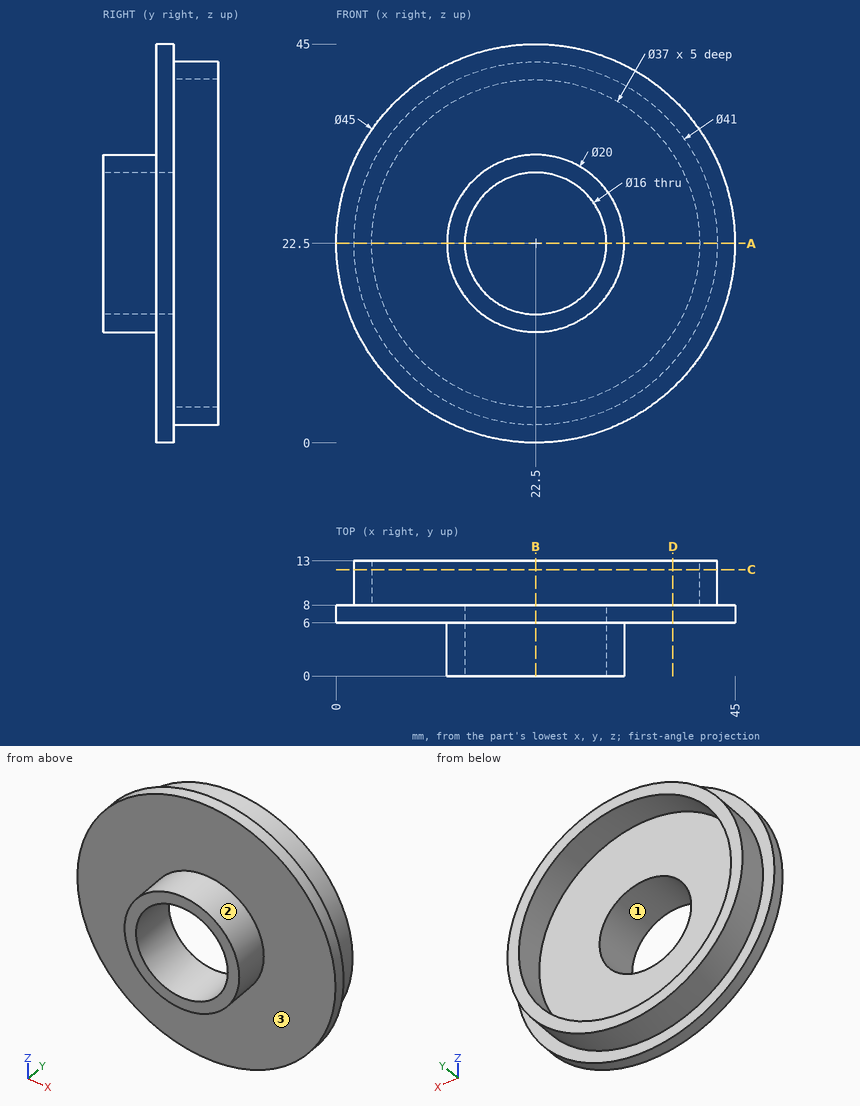
Input: dimensioned drawing with shaded views. Units: mm. Origin: part minimum x, y, z. Round coordinates to 2 decimals unless told otherwise and drop trailing zeros. Loops run counter-clockwise (first coordinate to the right, second up) from the corner with the lowest first, then second, coordinate; pieces in that order, holes last. Notation, with made-up numbers: (20.5, 1) -> (41.5, 1) arc R9 ccw to (41.5, 13) -> close; hole circle Ø4 at (-33, -23). An arc over 180 degrees is marked (long way). Answer as a JSON object with one key per item and string values. Group by question number.
1) Ray query, L1, parallel to Z at x = 22.5, y = 11.7; L2, parallel to Z at x = 22.5, y = 6.75. Return the intervals inside material, ascending.
2) Section query A-A on z = 22.5. Output: boundary loops of the cut face in (x, y).
3) Section query B-B on x = 22.5. Output: boundary loops of the cut face in (y, z).
4) Draft query along X for the marked faces 1, 2 and 3. Return one class per face: +X half, -X half, draft (parallel to the pull), parting line (faces both ways), or undercut.
5) Section query C-C on y = 12. Output: boundary loops of the cut face in (x, z), plus the area to 3 significant figures.
6) Pin query (flat end, axial travel): pin 1 (11 mm diameter, centred on x = 17, z = 26.5, fed in from +Y); pin 2 (5 mm diameter, centred on x = 9.5, z = 40, fed in from -Y); pin 3 (4 mm diameter, centred on y = 3.5, z = 20.5, fed in from -X). Return the tip coordinate at first contact, or that it passes through.
7) Section query D-D on x = 38. Output: boundary loops of the cut face in (y, z), plus the area to 3 significant figures.
Reply:
{
 "1": {"L1": "z = 2 to 4, 41 to 43", "L2": "z = 0 to 14.5, 30.5 to 45"},
 "2": {"outline": "(0, 6) -> (12.5, 6) -> (12.5, 0) -> (14.5, 0) -> (14.5, 8) -> (4, 8) -> (4, 13) -> (2, 13) -> (2, 8) -> (0, 8) -> close; (30.5, 0) -> (32.5, 0) -> (32.5, 6) -> (45, 6) -> (45, 8) -> (43, 8) -> (43, 13) -> (41, 13) -> (41, 8) -> (30.5, 8) -> close"},
 "3": {"outline": "(0, 12.5) -> (6, 12.5) -> (6, 0) -> (8, 0) -> (8, 2) -> (13, 2) -> (13, 4) -> (8, 4) -> (8, 14.5) -> (0, 14.5) -> close; (0, 30.5) -> (8, 30.5) -> (8, 41) -> (13, 41) -> (13, 43) -> (8, 43) -> (8, 45) -> (6, 45) -> (6, 32.5) -> (0, 32.5) -> close"},
 "4": {"face 1": "undercut", "face 2": "parting line", "face 3": "draft"},
 "5": {"outline": "circle Ø41 at (22.5, 22.5); hole circle Ø37 at (22.5, 22.5)", "area": "245 mm2"},
 "6": {"pin 1": "stops at y = 8", "pin 2": "stops at y = 6", "pin 3": "stops at x = 12.5"},
 "7": {"outline": "(6, 6.19) -> (8, 6.19) -> (8, 9.08) -> (13, 9.08) -> (13, 12.4) -> (8, 12.4) -> (8, 32.6) -> (13, 32.6) -> (13, 35.92) -> (8, 35.92) -> (8, 38.81) -> (6, 38.81) -> close", "area": "98.4 mm2"}
}
